Check sheet for the modelled part. Datum: model origin and axes. Units: mm. A direction names the side the tool comes from. Give positions to 0.01 mm unless a question says otherwise; leave off trailing zeros. Write each loop counter-clockwise with the first axis right and the second up, starting at its lowest first coordinate (ties: lowest second). Pieces come first, ordered by that corner, then holes.
from build123d import *

# Parameters (mm, degrees)
SKETCH1_W           = 135.25
SKETCH1_H           = 100
BOSS_EXTRUDE1_DEPTH = 22
SKETCH4_W           = 5
SKETCH4_H           = 19
CUT_EXTRUDE1_DEPTH  = 101
SKETCH5_W           = 117.25
SKETCH5_H           = 11
CUT_EXTRUDE2_DEPTH  = 101
FILLET1_R           = 10
FILLET2_R           = 10
FILLET3_R           = 10
FILLET4_R           = 10
FILLET5_R           = 10
SKETCH6_R           = 4
CUT_EXTRUDE3_DEPTH  = 136.25


with BuildPart() as part:
    # Sketch1 → Boss-Extrude1 (new body)
    with BuildSketch(Plane(origin=(0, 0, 0), x_dir=(1, 0, 0), z_dir=(0, 1, 0))):
        Rectangle(SKETCH1_W, SKETCH1_H)
    extrude(amount=BOSS_EXTRUDE1_DEPTH)

    # Sketch4 → Cut-Extrude1 (cut, through all)
    with BuildSketch(Plane.XY.offset(50)):
        with Locations((-61.125, 9.5)):
            Rectangle(SKETCH4_W, SKETCH4_H)
        with Locations((61.125, 9.5)):
            Rectangle(SKETCH4_W, SKETCH4_H)
    extrude(amount=-CUT_EXTRUDE1_DEPTH, mode=Mode.SUBTRACT)

    # Sketch5 → Cut-Extrude2 (cut, through all)
    with BuildSketch(Plane(origin=(0, 0, -50), x_dir=(-1, 0, 0), z_dir=(0, 0, -1))):
        Rectangle(SKETCH5_W, SKETCH5_H)
    extrude(amount=-CUT_EXTRUDE2_DEPTH, mode=Mode.SUBTRACT)

    # Fillet1
    fillet1_edges = [part.edges().sort_by_distance(p)[0] for p in [
        (0, 5.5, 50),
    ]]
    fillet(fillet1_edges, radius=FILLET1_R)

    # Fillet2
    fillet2_edges = [part.edges().sort_by_distance(p)[0] for p in [
        (-65.625, 0, 50),
    ]]
    fillet(fillet2_edges, radius=FILLET2_R)

    # Fillet3
    fillet3_edges = [part.edges().sort_by_distance(p)[0] for p in [
        (65.625, 0, 50),
    ]]
    fillet(fillet3_edges, radius=FILLET3_R)

    # Fillet4
    fillet4_edges = [part.edges().sort_by_distance(p)[0] for p in [
        (-65.625, 0, -50),
    ]]
    fillet(fillet4_edges, radius=FILLET4_R)

    # Fillet5
    fillet5_edges = [part.edges().sort_by_distance(p)[0] for p in [
        (65.625, 0, -50),
    ]]
    fillet(fillet5_edges, radius=FILLET5_R)

    # Sketch6 → Cut-Extrude3 (cut, through all)
    with BuildSketch(Plane.ZY.offset(67.625)):
        with Locations((-43, 13)):
            Circle(SKETCH6_R)
    extrude(amount=-CUT_EXTRUDE3_DEPTH, mode=Mode.SUBTRACT)


solid = part.part
1) Sectioned sample at D-D on z = 17.5. Record the boundary of the cut face in (x, y) (3 decimals).
2) Access from +Z, -Z, +X, -X, +Y, -Y to the whole of each face (thin tool, end or side, straight path). Record for faces 1 (the cylindrical face through (-65.6, 3.01, -47.15)), 2 (the flat face through (1, 5.5, -6)), 3 (the cylindrical face through (-0.82, 8.51, 47.15)).
3) Sectioned sample at A-A on y = 13. Record the boundary of the cut face in (x, z) (3 decimals), then the cut area to 3 significant figures.
4) Sectioned sample at C-C on x = 13. Record the boundary of the cut face in (y, z).
5) Draft check along Z on faces 4 (the cylindrical face through (65.65, 3.01, -47.15)), 5 (the cylindrical face through (-0.82, 15.7, -45.95)), 6 (the flat face through (-1, 19, 50)). Enter one of: +Z half, -Z half, draft (parallel to the pull), parting line (faces both ways), or undercut.
6) Scan lines: L1, parallel to X at y = 10, z = -1.5 (3 decimals); L2, parallel to X at y = 3, z = -8.5 (3 decimals); L3, parallel to Y at x = -4, z = -43. Record each from-to range of solid material in increasing order.
7) Sectioned sample at B-B on z = -43. Record the boundary of the cut face in (x, y) (3 decimals), then the cut area to 3 significant figures.
8) Gauge pin test, flat ends, axial feed: pin 1 (4 mm diameter, centred on x = 61.5, z = -7, fed in from -Y); pin 2 (5 mm diameter, centred on x = -49, z = 22, fed in from -Y). Record the tip position at first contact, or that the pin passes through.
Answers below:
1. outline: (-67.625, 0) - (-63.625, 0) - (-63.625, 19) - (-58.625, 19) - (-58.625, 5.5) - (58.625, 5.5) - (58.625, 19) - (63.625, 19) - (63.625, 0) - (67.625, 0) - (67.625, 22) - (-67.625, 22) - close
2. face 1: -Z, -X, -Y
2. face 2: +Z, -Z, -Y
2. face 3: +Z, -Y
3. outline: (-67.625, -50) - (-63.625, -50) - (-63.625, -47) - (-67.625, -47) - close; (-67.625, -39) - (-63.625, -39) - (-63.625, 50) - (-67.625, 50) - close; (-58.625, -50) - (58.625, -50) - (58.625, -47) - (-58.625, -47) - close; (-58.625, -39) - (58.625, -39) - (58.625, 49.682) - (-58.625, 49.682) - close; (63.625, -50) - (67.625, -50) - (67.625, -47) - (63.625, -47) - close; (63.625, -39) - (67.625, -39) - (67.625, 50) - (63.625, 50) - close
3. area: 11,500 mm2
4. outline: (5.5, -50) - (22, -50) - (22, 50) - (15.5, 50) arc R10 ccw to (5.5, 40) - close; hole circle Ø8 at (13, -43)
5. face 4: -Z half
5. face 5: undercut
5. face 6: +Z half
6. L1: x = -67.625 to -63.625, -58.625 to 58.625, 63.625 to 67.625
6. L2: x = -67.625 to -63.625, 63.625 to 67.625
6. L3: y = 5.5 to 9, 17 to 22
7. outline: (-67.625, 0.461) - (-63.625, 0.461) - (-63.625, 9) - (-67.625, 9) - close; (-67.625, 17) - (-63.625, 17) - (-63.625, 19) - (-58.625, 19) - (-58.625, 17) - (58.625, 17) - (58.625, 19) - (63.625, 19) - (63.625, 17) - (67.625, 17) - (67.625, 22) - (-67.625, 22) - close; (-58.625, 5.5) - (58.625, 5.5) - (58.625, 9) - (-58.625, 9) - close; (63.625, 0.461) - (67.625, 0.461) - (67.625, 9) - (63.625, 9) - close
7. area: 1,130 mm2
8. pin 1: stops at y = 19
8. pin 2: stops at y = 5.5
